Study the drawing (mm; zero at the part's minimum x, y, z) and answer. Coordinates: 2 decimals unless noted, no trailing zeros. Order: outer loops, then holes, each group sorted by start corner. A loop starts at its lowest first (then second) coordinate and runs counter-clockwise, first axis right, second up.
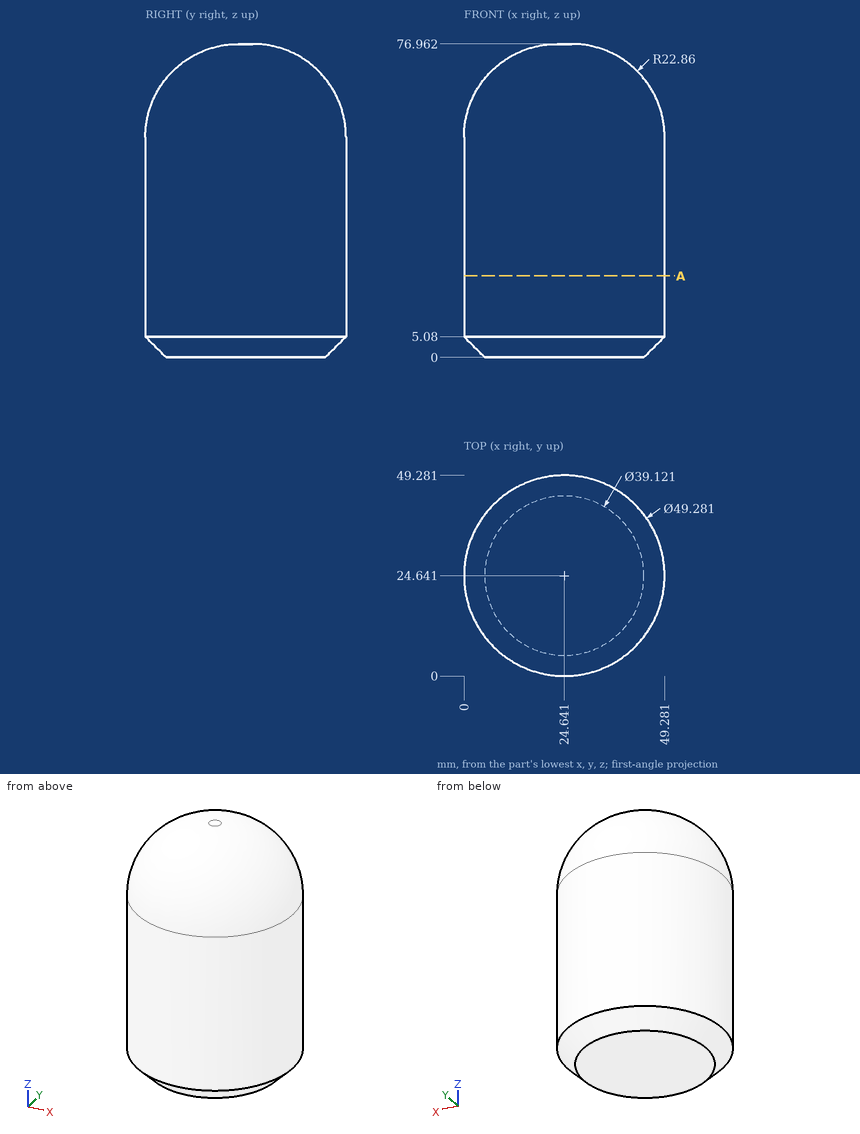
1) Straight lines are drawn through the part: line 1 (X direction, y = 24, z = 41); line 2 (Z direction, x = 26, y = 43.5) (1 decimal); line 3 (Y direction, x = 17.5, z = 46) (1 decimal). For each, find the intervals that lie inside material, in ascending order.
A:
line 1: x = 0.01 to 49.27
line 2: z = 0 to 69.2
line 3: y = 1.1 to 48.2
2) A cutting plane is placed at A-A, the plane z = 20. Determine the outline of the cut face in (x, y), and give its area (3 significant figures).
A:
outline: circle Ø49.28 at (24.64, 24.64)
area: 1,910 mm2
3) Flat-ended cylindrical pins translate along their axes: pin 1 Ø4 at (y, z) = (37, 32.5) entering from -X; pin 2 Ø1 at (x, z) = (37.5, 54.5) entering from +Y (1 decimal); pin 3 Ø1 at (x, z) = (23.5, 45) entering from -Y; pin 4 Ø6 at (x, y) = (23.5, 27.5) entering from +Z. Find the tip coordinate at first contact, or state that the pin passes through.
A:
pin 1: stops at x = 2.28
pin 2: stops at y = 46
pin 3: stops at y = 0.01
pin 4: stops at z = 76.96
